For this review, use the dimensioned drawing (mm, ordinates from the lowest corner) and the shaded views. A direction names the side the tool comes from. Coordinates: 2 decimals unless noted, no trailing zeros. Write each loop counter-clockwise with the first axis right and the second up, starting at its lowest first coordinate (ties: lowest second). Pieces come first, ordered by that corner, then holes. Notation, with made-up numbers: (5.25, 30.5) -> (56.25, 30.5) arc R27 ccw to (56.25, 50.5) -> close; hole circle Ø7 at (42.5, 35). An arc over 180 degrees is marked (long way). Put each result on its own line as item: value. Start each with the question number.
Item 1: For the marked faces 1 and 2, list the 3-axis set-ups (+Z, -Z, +X, -X, +Y, -Y) from which the entire face can be reached by the end or side of a thin tool; tool diameter is ignored.
Item 2: Consider section D-D on x = 11. Give the boundary of the cut face in (y, z).
Item 3: Consider section B-B on x = 29. Give the boundary of the cut face in (y, z).
Item 4: Consider section C-C on z = 3.5. Give the boundary of the cut face in (x, y).
Item 5: To check wall thickness, follow L1, parallel to Z at x = 25, y = 9; L2, parallel to Z at x = 23.5, y = 14.25. State the ranges of each line that lie inside material, in increasing order.
Item 6: Consider section A-A on y = 11.25. Give the boundary of the cut face in (x, z), and give its area (3 significant figures).
Item 7: Insertion check: P1, Ø3, axis at x = 26, z = 14.5, coming from the +Y side; P2, Ø12, axis at x = 31, y = 4, coming from the -Z side; P3, Ø2, axis at y = 11.5, z = 4.5, coming from the +X side; P4, Ø3, axis at x = 25.5, y = 16, coming from the +Z side. Each pin has a flat end and moves straight along its axis. Give the tip position at first contact, or say it passes through.
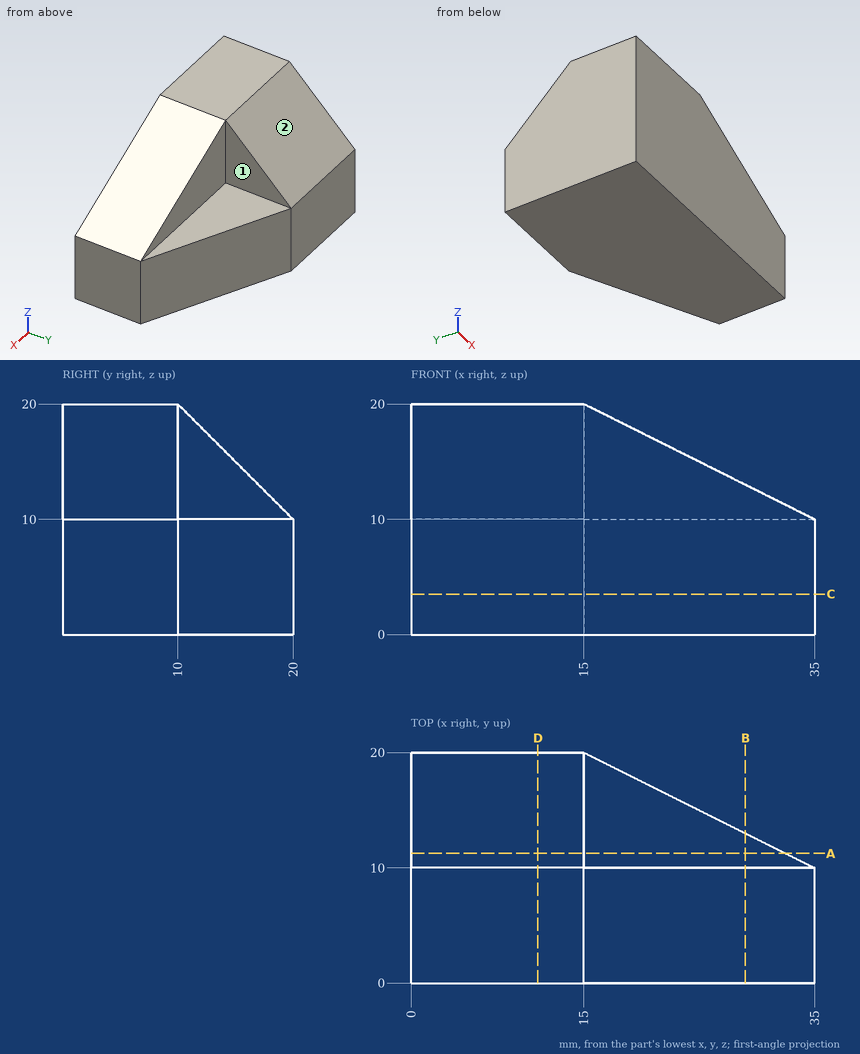
Return value:
1. face 1: +Z, +X, +Y
1. face 2: +Z, +X, -X, +Y
2. outline: (0, 0) -> (20, 0) -> (20, 10) -> (10, 20) -> (0, 20) -> close
3. outline: (0, 0) -> (13, 0) -> (13, 10) -> (10, 10) -> (10, 13) -> (0, 13) -> close
4. outline: (0, 0) -> (35, 0) -> (35, 10) -> (15, 20) -> (0, 20) -> close
5. L1: 0 to 15
5. L2: 0 to 10
6. outline: (0, 0) -> (32.5, 0) -> (32.5, 10) -> (15, 10) -> (15, 18.75) -> (0, 18.75) -> close
6. area: 456 mm^2
7. P1: y = 10
7. P2: z = 0
7. P3: x = 34
7. P4: z = 10
